Autodesk Inventor part; units mm, degrees
ref_plane "YZ Plane" through (0, 0, 0) normal (1, 0, 0) x (0, 1, 0)
ref_plane "XZ Plane" through (0, 0, 0) normal (0, 1, 0) x (-1, 0, 0)
ref_plane "XY Plane" through (0, 0, 0) normal (0, 0, 1) x (1, 0, 0)
sketch "Sketch1" plane through (0, 0, 0) normal (0, 1, 0) x (-1, 0, 0)
  line L0 (0, 0) -> (4.445, 0)
  line L1 (0, 0) -> (0, -3.175)
  line L2 (0, -3.175) -> (-3.175, -3.175)
  line L3 (-3.175, -3.175) -> (-3.175, 0)
  line L4 (-3.175, 0) -> (-7.62, 0)
  line L5 (-7.62, 0) -> (-7.62, -3.175)
  line L6 (-7.62, -3.175) -> (-10.795, -3.175)
  line L7 (-10.795, -3.175) -> (-10.795, 0)
  line L8 (-10.795, 0) -> (-15.24, 0)
  line L9 (-15.24, 0) -> (-15.24, -12.7)
  line L10 (-15.24, -12.7) -> (4.445, -12.7)
  line L11 (4.445, -12.7) -> (4.445, 0)
  line L12 (-15.24, 0) -> (-15.24, -50.8) construction
  line L13 (-15.24, -50.8) -> (-2.54, -50.8) construction
  dimension "d0" = 4.445
  dimension "d1" = 3.175
  dimension "d2" = 3.175
  dimension "d3" = 4.445
  dimension "d4" = 3.175
  dimension "d5" = 4.445
  dimension "d6" = 12.7
  dimension "d7" = 50.8
  dimension "d36" = 12.7
  dimension "d38" = 12.7
revolve "Revolution1" add sketch "Sketch1" angle 360 about axis through (15.24, 0, -50.8) along (-1, 0, 0)
sketch "Sketch2" plane through (-4.445, 0, -50.8) normal (-1, 0, 0) x (0, 0, 1)
  circle A0 centre (0, 0) radius 38.1
  circle A1 centre (0, 0) radius 63.5
  circle A2 centre (0, 0) radius 38.1
  dimension "d9" = 76.2
  dimension "d10" = 127
extrude "Extrusion1" add sketch "Sketch2" along normal blind 6.096
sketch "Sketch3" plane through (-10.541, 0, -50.8) normal (-1, 0, 0) x (0, 0, 1)
  circle A0 centre (0, 0) radius 49.0093
  circle A1 centre (0, 0) radius 52.1843
  circle A2 centre (0, 0) radius 38.1
  dimension "d41" = 10.9093
  dimension "d42" = 3.175
extrude "Extrusion2" cut sketch "Sketch3" against normal blind 3.5306 contours A1
chamfer "Chamfer1" distance 1.778 angle 45 1 edges at (15.24, 0, -101.6)
sketch "Sketch5" plane through (-10.541, 0, -50.8) normal (-1, 0, 0) x (0, 0, 1)
  circle A0 centre (0, 0) radius 55.245 construction
  circle A1 centre (0, 0) radius 38.1
  point P0 (-55.245, 0)
  point P1 (-27.6225, -47.8436)
  point P2 (27.6225, -47.8436)
  point P3 (55.245, 0)
  point P4 (27.6225, 47.8436)
  point P5 (-27.6225, 47.8436)
  dimension "d43" = 110.49
  dimension "d46" = 360
hole "Hole1" at (-10.541, 0, -106.045) at (-10.541, -47.8436, -78.4225) at (-10.541, -47.8436, -23.1775) at (-10.541, 0, 4.445) at (-10.541, 47.8436, -23.1775) at (-10.541, 47.8436, -78.4225) direction (1, 0, 0) diameter 3.5052 end through all
chamfer "Chamfer2" distance 0.254 angle 45 6 edges at (0, 0, -101.6) (3.175, 0, -101.6) (7.62, 0, -101.6) (10.795, 0, -101.6) (-10.541, 0, -102.9843) (-10.541, 0, -99.8093)
properties part number "Oring Fitting Dome V3"
Build history of the part. All positions in model axes, mm. A direction names the side the tool comes from. Give positions to 0.01 mm unless a question says otherwise; leave off trailing zeros.
1) Two-plate mould, pull along X, no slides. Class faces 4 (the face through (3.175, 34, -85)), 5 (the face through (-8.672, -18.771, -5.528)), 6 (the face through (7.62, 34, -85)), 7 (the face through (-4.445, 43, -79)): released by +X, released by -X, zero draft, split by the parting line, or undercut.
Values follow:
face 4: undercut
face 5: zero draft
face 6: undercut
face 7: released by +X
2) 3-axis set-ups, long thin cutter, end or side, ignore diameter. For faces 1 (the face through (0, 34, -85)), 2 (the face through (-7.01, 47, -36)), 3 (the face through (-2.379, 15.259, -2.346)): which of +Z, -Z, +X, -X, +Y, -Y reach the whole face in a straight line?
Values follow:
face 1: none
face 2: -X
face 3: +X
3) Band-saw the part on A-A on y = 0. State how many separate pieces and enclosed holes the cut face has, then the cut area to 3 significant figures.
Values follow:
separate pieces: 4
enclosed holes: 0
area: 701 mm2
4) Drop flat-ended pins along their axis: P1, Ø4, axis at x = -4, y = 29, coming from the +Z side; P2, Ø1, axis at x = 11.5, y = -39, coming from the -Z side; P3, Ø4, axis at y = -47.84, z = -23.18, coming from the +X side (3 decimals). Give the stop position or say it passes through.
Values follow:
P1: stops at z = 6.65
P2: stops at z = -83.94
P3: stops at x = -4.445
5) Probe line 1 along Z through (x, y) = (9, -0.5); line 2 along X through (y, z) = (51.5, -67) (3 decimals); line 3 along Z through (x, y) = (0.75, 28.5). List the from-to ranges inside material, lowest first.
Values follow:
line 1: z = -98.42 to -88.9, -12.7 to -3.18
line 2: x = -10.541 to -4.445
line 3: z = -88.96 to -76.09, -25.51 to -12.64
